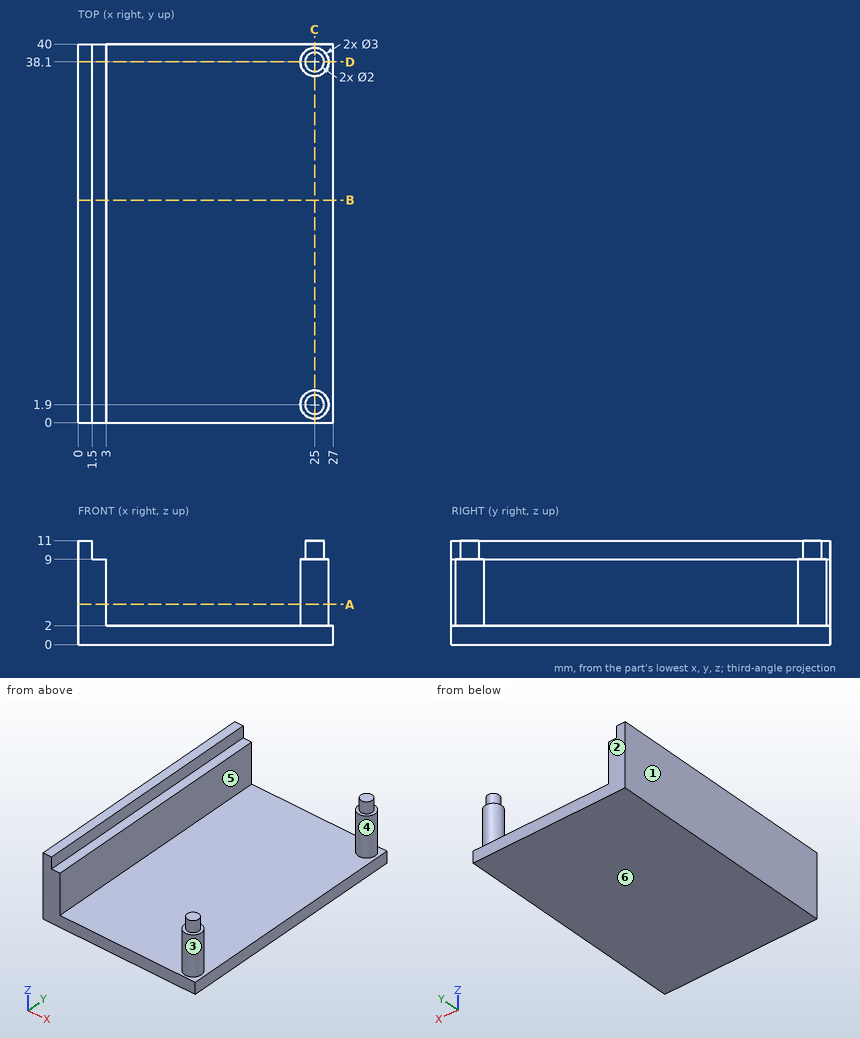
Drawing for the job (mm, zero at the part's lowest x, y, z). A direction names the side the tool comes from. Round coordinates to 2 decimals unless told otherwise and drop trailing zeros. Order: outer loops, then holes, each group sorted by start corner. A loop starts at its lowest first (then second) coordinate and runs counter-clockwise, first axis right, second up.
Item 1: Saw through at A-A on z = 4.25. Write the cut outline in (x, y).
Item 2: Saw through at B-B on y = 23.5. Write the cut outline in (x, z), then the cut area to 3 significant figures.
Item 3: Pin check, flat tips, straight feed: pin 1 (1 mm diameter, centred on y = 9, z = 4.5, fed in from +X); pin 2 (1.6 mm diameter, centred on x = 2.5, y = 12, fed in from +Z); pin 3 (1.6 mm diameter, centred on y = 22, z = 10, fed in from +X). Stop position of each tip, or through.
Item 4: Tool access for the marked faces 4, 5 and 6: list every direction of +Z, -Z, +X, -X, +Y, -Y with a clear straight run to the whole face (end or side of a thin tool).
Item 5: Saw through at C-C on x = 25. Write the cut outline in (y, z), then the cut area to 3 significant figures.
Item 6: Probe line 1 along Z through (x, y) = (15.75, 38); line 2 along X through (y, z) = (4.5, 5.5); line 3 along X through (y, z) = (7.5, 9.25). List the from-to ranges inside material, lowest first.
Item 7: Mould opens along Y. For the marked faces 1, 2 and 3 say: pulls with the +Y half, pulls with the -Y half, needs draft (parallel to the pull), parting line crosses it, or undercut.
Item 8: Saw through at D-D on y = 38.1. Write the cut outline in (x, z), then the cut area to 3 significant figures.
Reported:
1. outline: (0, 0) - (3, 0) - (3, 40) - (0, 40) - close; circle Ø3 at (25, 1.9); circle Ø3 at (25, 38.1)
2. outline: (0, 0) - (27, 0) - (27, 2) - (3, 2) - (3, 9) - (1.5, 9) - (1.5, 11) - (0, 11) - close
2. area: 78.0 mm2
3. pin 1: stops at x = 3
3. pin 2: stops at z = 9
3. pin 3: stops at x = 1.5
4. face 4: +Z
4. face 5: +Z, +Y, -Y
4. face 6: -Z, +X, -X, +Y, -Y
5. outline: (0, 0) - (40, 0) - (40, 2) - (39.6, 2) - (39.6, 9) - (39.1, 9) - (39.1, 11) - (37.1, 11) - (37.1, 9) - (36.6, 9) - (36.6, 2) - (3.4, 2) - (3.4, 9) - (2.9, 9) - (2.9, 11) - (0.9, 11) - (0.9, 9) - (0.4, 9) - (0.4, 2) - (0, 2) - close
5. area: 130 mm2
6. line 1: z = 0 to 2
6. line 2: x = 0 to 3
6. line 3: x = 0 to 1.5
7. face 1: needs draft
7. face 2: pulls with the +Y half
7. face 3: undercut
8. outline: (0, 0) - (27, 0) - (27, 2) - (26.5, 2) - (26.5, 9) - (26, 9) - (26, 11) - (24, 11) - (24, 9) - (23.5, 9) - (23.5, 2) - (3, 2) - (3, 9) - (1.5, 9) - (1.5, 11) - (0, 11) - close
8. area: 103 mm2
